Geometry: final body of the model. Coordinates: model frame, mm. A direction names the side the tool comes from. Give positions to 0.01 mm unless a question says otherwise; leave off trailing zeros. Loops run counter-clockwise (first coordinate to the right, second up) from the corner with the lowest first, then second, coordinate; pieces in that order, holes last.
1. Section B-B, the plane x = -4.25. Output: boundary loops of the cut face in (y, z).
2. Section C-C, the plane y = 5. Output: boundary loops of the cut face in (x, z).
3. Material intervals for line 1 along Y through (x, z) = (0, 4.5); line 2 along Y through (x, z) = (-4.25, 4.25); line 3 along Z through (x, y) = (5, 6.25), sorted ascending.
4. Draft query along Y for faces 1 (the face through (-1.5, 5.07, 5.18)), 2 (the face through (-5.699, 8.715, 5.07)), 3 (the face through (-5.699, -8.715, 5.07)). Return one class per face: +Y half, -Y half, draft (parallel to the pull), parting line (faces both ways), or undercut.
5. Access query for faces 4 (the face through (-0.26, 6.983, 10.246)), 5 (the face through (5.715, -8.699, 5.07)). Directions: +Z, -Z, +X, -X, +Y, -Y. A direction counts if a zero-diameter tool reaches every point of the face in a straight line with its end or side. Return the directions, or none.
6. First-contact query: P1, Ø0.8, axis at x = -4.25, y = 7.25, coming from the -Z side; P2, Ø3.5, axis at x = -3, y = -2, coming from the +Z side. Flat tips, straight axial feed; report the tip coordinate or a pass-through.
7. Section D-D, the plane z = 9. Output: boundary loops of the cut face in (x, y).
8. Section A-A, the plane y = 7.25. Output: boundary loops of the cut face in (x, z).
from build123d import *

# Parameters (mm, degrees)
SKETCH_1_W      = 12
SKETCH_1_H      = 18
SKETCH_1_R      = 1.5
SKETCH_1_R_2    = 0.7
EXTRUDE_1_DEPTH = 10
SKETCH_2_R      = 2
SKETCH_2_R_2    = 1.5
EXTRUDE_2_DEPTH = 0.5
FILLET_1_R      = 1


with BuildPart() as part:
    # 草图1 → 凸台-拉伸1 (new body)
    with BuildSketch(Plane.XY):
        Rectangle(SKETCH_1_W, SKETCH_1_H)
        with Locations((0, 5)):
            Circle(SKETCH_1_R, mode=Mode.SUBTRACT)
        with Locations((-4.25, 7.25)):
            Circle(SKETCH_1_R_2, mode=Mode.SUBTRACT)
        with Locations(Location((4.25, 7.25, 0), (0, 0, 180))):
            Circle(SKETCH_1_R_2, mode=Mode.SUBTRACT)
    extrude(amount=EXTRUDE_1_DEPTH)

    # 草图2 → 凸台-拉伸2 (add)
    with BuildSketch(Plane.XY.offset(10)):
        with Locations((0, 5)):
            Circle(SKETCH_2_R)
        with Locations((0, 5)):
            Circle(SKETCH_2_R_2, mode=Mode.SUBTRACT)
    extrude(amount=EXTRUDE_2_DEPTH)

    # 圆角1
    fillet_1_edges = [part.edges().sort_by_distance(p)[0] for p in [
        (-6, 9, 5),
        (6, 9, 5),
        (6, -9, 5),
        (-6, -9, 5),
    ]]
    fillet(fillet_1_edges, radius=FILLET_1_R)


solid = part.part
Answers below:
1. outline: (-9, 0) - (6.55, 0) - (6.55, 10) - (-9, 10) - close; (7.95, 0) - (9, 0) - (9, 10) - (7.95, 10) - close
2. outline: (-6, 0) - (-1.5, 0) - (-1.5, 10.5) - (-2, 10.5) - (-2, 10) - (-6, 10) - close; (1.5, 0) - (6, 0) - (6, 10) - (2, 10) - (2, 10.5) - (1.5, 10.5) - close
3. line 1: y = -9 to 3.5, 6.5 to 9
3. line 2: y = -9 to 6.55, 7.95 to 9
3. line 3: z = 0 to 10
4. face 1: undercut
4. face 2: +Y half
4. face 3: -Y half
5. face 4: +Z
5. face 5: +Z, -Z, +X, -Y
6. P1: passes through
6. P2: stops at z = 10
7. outline: (-6, -8) arc R1 ccw to (-5, -9) - (5, -9) arc R1 ccw to (6, -8) - (6, 8) arc R1 ccw to (5, 9) - (-5, 9) arc R1 ccw to (-6, 8) - close; hole circle Ø1.4 at (-4.25, 7.25); hole circle Ø3 at (0, 5); hole circle Ø1.4 at (4.25, 7.25)
8. outline: (-6, 0) - (-4.95, 0) - (-4.95, 10) - (-6, 10) - close; (-3.55, 0) - (3.55, 0) - (3.55, 10) - (-3.55, 10) - close; (4.95, 0) - (6, 0) - (6, 10) - (4.95, 10) - close
